The model under review builds one solid part; all positions refer to its coordinate system, in mm. Round coordinates to 2 decimals unless told otherwise and drop trailing zeros. Loops run counter-clockwise (first coordinate to the right, second up) from the corner with the lowest first, then second, coordinate; pieces in that order, holes last. Notation, with made-up numbers: (-29.5, 8.25) -> (23.5, 8.25) arc R30 ccw to (23.5, 44.25) -> close; hole circle Ø9 at (31, -18.75). An arc over 180 degrees is marked (long way). Use a Markdown table: item, result. Add a question column.
1) Insertion check: pin 1 (2.5 mm diameter, centred on x = -103.59, y = -2.81, fed in from -Z). The pin has a flat end and moves straight along its axis. Give the tip position at first contact, or say it passes through.
2) Consider section B-B on x = -1.5. Give the boundary of the cut face in (y, z).
3) Consider section A-A on z = 0.1. State how many separate pieces and enclosed holes the cut face has, plus the area to 3 significant figures.
4) Wall thickness on probe 1 along Y at (x, z) = (-97.5, 0.1); probe 2 along Y at (x, z) = (-102.5, 0.25): over which ranges is each line inside the solid? List them lowest first.
from build123d import *

# Parameters (mm, degrees)
F0_W     = 178
F0_H     = 30
F0_R     = 1.6
F1_DEPTH = 0.282222


with BuildPart() as f1:
    # F0 (on Top) → F1 (new body)
    with BuildSketch(Plane.XY):
        with Locations((-39.587713, 7.19178)):
            Rectangle(F0_W, F0_H)
        with Locations((-123.356734, -2.80822)):
            Circle(F0_R, mode=Mode.SUBTRACT)
        with Locations((-103.587713, -2.80822)):
            Circle(F0_R, mode=Mode.SUBTRACT)
        with Locations((-97.587713, -2.80822)):
            Circle(F0_R, mode=Mode.SUBTRACT)
        with Locations((-77.587713, -2.80822)):
            Circle(F0_R, mode=Mode.SUBTRACT)
        with Locations((-62.587713, -2.80822)):
            Circle(F0_R, mode=Mode.SUBTRACT)
        with Locations((-42.587713, -2.80822)):
            Circle(F0_R, mode=Mode.SUBTRACT)
        with Locations((-36.587713, -2.80822)):
            Circle(F0_R, mode=Mode.SUBTRACT)
        with Locations((-16.587713, -2.80822)):
            Circle(F0_R, mode=Mode.SUBTRACT)
        with Locations((-1.587713, -2.80822)):
            Circle(F0_R, mode=Mode.SUBTRACT)
        with Locations((18.412287, -2.80822)):
            Circle(F0_R, mode=Mode.SUBTRACT)
        with Locations((24.412287, -2.80822)):
            Circle(F0_R, mode=Mode.SUBTRACT)
        with Locations((44.412287, -2.80822)):
            Circle(F0_R, mode=Mode.SUBTRACT)
        with Locations((-123.587713, 17.19178)):
            Circle(F0_R, mode=Mode.SUBTRACT)
        with Locations((-103.587713, 17.19178)):
            Circle(F0_R, mode=Mode.SUBTRACT)
        with Locations((-97.587713, 17.19178)):
            Circle(F0_R, mode=Mode.SUBTRACT)
        with Locations((-77.587713, 17.19178)):
            Circle(F0_R, mode=Mode.SUBTRACT)
        with Locations((-62.587713, 17.19178)):
            Circle(F0_R, mode=Mode.SUBTRACT)
        with Locations((-42.587713, 17.19178)):
            Circle(F0_R, mode=Mode.SUBTRACT)
        with Locations((-36.587713, 17.19178)):
            Circle(F0_R, mode=Mode.SUBTRACT)
        with Locations((-16.587713, 17.19178)):
            Circle(F0_R, mode=Mode.SUBTRACT)
        with Locations((-1.587713, 17.19178)):
            Circle(F0_R, mode=Mode.SUBTRACT)
        with Locations((18.412287, 17.19178)):
            Circle(F0_R, mode=Mode.SUBTRACT)
        with Locations((24.412287, 17.19178)):
            Circle(F0_R, mode=Mode.SUBTRACT)
        with Locations((44.412287, 17.19178)):
            Circle(F0_R, mode=Mode.SUBTRACT)
    extrude(amount=F1_DEPTH)


solid = f1.part
Result set:
| question | item | result |
|---|---|---|
| 1 | pin 1 | through |
| 2 | outline | (-7.81, 0) -> (-4.41, 0) -> (-4.41, 0.28) -> (-7.81, 0.28) -> close; (-1.21, 0) -> (15.59, 0) -> (15.59, 0.28) -> (-1.21, 0.28) -> close; (18.79, 0) -> (22.19, 0) -> (22.19, 0.28) -> (18.79, 0.28) -> close |
| 3 | separate pieces | 1 |
| 3 | enclosed holes | 24 |
| 3 | area | 5,150 mm2 |
| 4 | probe 1 | -7.81 to -4.41, -1.21 to 15.59, 18.79 to 22.19 |
| 4 | probe 2 | -7.81 to -3.98, -1.63 to 16.02, 18.37 to 22.19 |
